Read the model definition and answer for the solid it produces. Units are mm, in the model's axes. A direction names the side the tool comes from. Give positions to 0.01 mm unless a question says otherwise; leave off trailing zeros. Order: outer loops, then holes, each group sorted by start corner. A loop starts at its lowest first (then second) coordinate and runs counter-clockwise, first axis right, second up. Notation, with made-up numbers: M -20,85.25 L 7,85.25 A19 ccw 7,105.25 Z; hole C 34.25,18.5 d6. An arc over 180 degrees is marked long. One line per item, written item: value.
from build123d import *

# Parameters (mm, degrees)
SKETCH1_W           = 100
SKETCH1_H           = 100
BOSS_EXTRUDE1_DEPTH = 100
SKETCH3_R           = 15
CUT_EXTRUDE1_DEPTH  = 10
SKETCH5_R           = 10
CUT_EXTRUDE2_DEPTH  = 10
SKETCH8_R           = 13
CUT_EXTRUDE3_DEPTH  = 10
SKETCH12_R          = 12.5
CUT_EXTRUDE4_DEPTH  = 10
CUT_EXTRUDE5_START  = -10
SKETCH13_R          = 10
CUT_EXTRUDE5_DEPTH  = 10
SKETCH14_R          = 10
CUT_EXTRUDE6_DEPTH  = 10


with BuildPart() as part:
    # Sketch1 → Boss-Extrude1 (new body)
    with BuildSketch(Plane(origin=(0, 0, 0), x_dir=(1, 0, 0), z_dir=(0, 1, 0))):
        Rectangle(SKETCH1_W, SKETCH1_H)
    extrude(amount=BOSS_EXTRUDE1_DEPTH)

    # Sketch3 → Cut-Extrude1 (cut)
    with BuildSketch(Plane(origin=(0, 100, 0), x_dir=(1, 0, 0), z_dir=(0, 1, 0))):
        with Locations(Location((0, 0, 0), (0, 0, 270))):
            Circle(SKETCH3_R)
    extrude(amount=-CUT_EXTRUDE1_DEPTH, mode=Mode.SUBTRACT)

    # Sketch5 → Cut-Extrude2 (cut)
    with BuildSketch(Plane.XY.offset(50)):
        with Locations((0, 50)):
            Circle(SKETCH5_R)
        with Locations((24.748737342, 74.748737342)):
            Circle(SKETCH5_R)
        with Locations((-24.748737342, 25.251262658)):
            Circle(SKETCH5_R)
    extrude(amount=-CUT_EXTRUDE2_DEPTH, mode=Mode.SUBTRACT)

    # Sketch8 → Cut-Extrude3 (cut)
    with BuildSketch(Plane.ZY.offset(50)):
        with Locations((-16.970562748, 66.970562748)):
            Circle(SKETCH8_R)
        with Locations((16.970562748, 33.029437252)):
            Circle(SKETCH8_R)
    extrude(amount=-CUT_EXTRUDE3_DEPTH, mode=Mode.SUBTRACT)

    # Sketch12 → Cut-Extrude4 (cut)
    with BuildSketch(Plane(origin=(50, 0, 0), x_dir=(0, 0, -1), z_dir=(1, 0, 0))):
        with Locations((-25, 75)):
            Circle(SKETCH12_R)
        with Locations((25, 75)):
            Circle(SKETCH12_R)
        with Locations((25, 25)):
            Circle(SKETCH12_R)
        with Locations((-25, 25)):
            Circle(SKETCH12_R)
    extrude(amount=-CUT_EXTRUDE4_DEPTH, mode=Mode.SUBTRACT)

    # Sketch13 → Cut-Extrude5 (cut)
    with BuildSketch(Plane(origin=(0, 0, -50), x_dir=(-1, 0, 0), z_dir=(0, 0, -1)).offset(CUT_EXTRUDE5_START)):
        with Locations(Location((0, 50, 0), (0, 0, 180))):
            Circle(SKETCH13_R)
        with Locations((-27.5, 77.5)):
            Circle(SKETCH13_R)
        with Locations((27.5, 77.5)):
            Circle(SKETCH13_R)
        with Locations((27.5, 22.5)):
            Circle(SKETCH13_R)
        with Locations((-27.5, 22.5)):
            Circle(SKETCH13_R)
    extrude(amount=CUT_EXTRUDE5_DEPTH, mode=Mode.SUBTRACT)

    # Sketch14 → Cut-Extrude6 (cut)
    with BuildSketch(Plane(origin=(0, 0, 0), x_dir=(-1, 0, 0), z_dir=(0, -1, 0))):
        with Locations(Location((-16.67, 0, 0), (0, 0, 90))):
            Circle(SKETCH14_R)
        with Locations(Location((16.67, 0, 0), (0, 0, 90))):
            Circle(SKETCH14_R)
        with Locations(Location((16.67, 25, 0), (0, 0, 90))):
            Circle(SKETCH14_R)
        with Locations(Location((-16.67, 25, 0), (0, 0, 90))):
            Circle(SKETCH14_R)
        with Locations(Location((-16.67, -25, 0), (0, 0, 90))):
            Circle(SKETCH14_R)
        with Locations(Location((16.67, -25, 0), (0, 0, 90))):
            Circle(SKETCH14_R)
    extrude(amount=-CUT_EXTRUDE6_DEPTH, mode=Mode.SUBTRACT)


solid = part.part
1) Find section B-B, the plane y = 94. Write down the section's boundary in (x, z), plus the area to 3 significant figures.
Reported:
outline: M -50,-50 L 50,-50 L 50,50 L -50,50 Z; hole C 0,0 d30
area: 9,290 mm^2
2) Determine the mould class of faces 5 (the face through (-40, 33, 17)), 6 (the face through (17, 10, -25)), 7 (the face through (-8.24, 4.93, -5.38)) for opening direction Y: +Y half, -Y half, draft (parallel to the pull), parting line (faces both ways), or undercut.
Reported:
face 5: undercut
face 6: -Y half
face 7: draft
3) Find section A-A, the plane x = 44.5. Write down the section's boundary in (y, z).
Reported:
outline: M 0,-50 L 100,-50 L 100,50 L 0,50 Z; hole C 25,-25 d25; hole C 25,25 d25; hole C 75,-25 d25; hole C 75,25 d25
4) Which of the six approach directions +Z, -Z, +X, -X, +Y, -Y give full straight-line access (tool end or side, diameter ignored) to faces 1 (the face through (40, 25, 25)), 2 (the face through (-17, 10, 25)), 3 (the face through (-32.12, 32.01, 45.07)), 4 (the face through (-45.07, 79.86, -18.66))?
Reported:
face 1: +X
face 2: -Y
face 3: +Z
face 4: -X
5) Each of these flat-tipped pins is pushed along its axis until it touches: pin 1 Ø6 at (x, z) = (-14.5, 29) entering from -Y; pin 2 Ø10 at (x, y) = (-26, 77.5) entering from -Z; pin 3 Ø15.5 at (y, z) = (33.03, 16.97) entering from -X. Where does it stop, or does it pass through?
Reported:
pin 1: stops at y = 10
pin 2: stops at z = -40
pin 3: stops at x = -40
6) Find section C-C, the plane z = 0. Write down the section's boundary in (x, y).
Reported:
outline: M -50,0 L -26.67,0 L -26.67,10 L -6.67,10 L -6.67,0 L 6.67,0 L 6.67,10 L 26.67,10 L 26.67,0 L 50,0 L 50,100 L 15,100 L 15,90 L -15,90 L -15,100 L -50,100 Z
7) Find section D-D, the plane x = 5. Write down the section's boundary in (y, z).
Reported:
outline: M 0,-50 L 41.34,-50 L 41.34,-40 L 58.66,-40 L 58.66,-50 L 100,-50 L 100,-14.14 L 90,-14.14 L 90,14.14 L 100,14.14 L 100,50 L 58.66,50 L 58.66,40 L 41.34,40 L 41.34,50 L 0,50 Z
8) Consider probe 1 along X at (y, z) = (4.5, -25); probe 2 along Y at (x, z) = (27.5, -46.5); probe 3 along Z at (x, y) = (45, 73.5). Determine where each line is inside the solid, lowest interval first.
Reported:
probe 1: x = -50 to -26.67, -6.67 to 6.67, 26.67 to 50
probe 2: y = 0 to 12.5, 32.5 to 67.5, 87.5 to 100
probe 3: z = -50 to -37.41, -12.59 to 12.59, 37.41 to 50
